Geometry: final body of the model. Coordinates: model frame, mm. Coordinates: 2 decimals unless noted, no trailing zeros. Order: outer loops, then holes, each group sorted by start corner. A loop starts at its lowest first (then second) coordinate and runs counter-clockwise, first axis right, second up. Notation, with made-up numbers: (31.25, 29) -> (62.25, 29) arc R24 ccw to (62.25, 39) -> close; hole circle Ø7 at (87, 58). An arc over 180 degrees is marked (long way). Answer in a Markdown table with one row per item. Add a question column.
1) Contact query for flat-ended pins moving along their axis: P1, Ø3, axis at x = -1.5, z = 134.5, coming from the +Y side; P2, Ø5, axis at x = -1, z = 131, coming from the -Y side; P3, Ø3, axis at x = 0, z = -23, coming from the -Y side; P4, Ø4, axis at x = 2.5, y = 10.5, coming from the +Z side. Output: stop coordinate, or through.
2) Ray query, line 1 (Y direction, x = 0, z = -0.25); line 2 (X direction, y = 22, z = 58.5); line 3 (Y direction, x = 0, z = 117.5). Return the intervals inside material, ascending. Write a range as from..to.
3) Section query A-A on z = 84. Return the cut outline in (x, y).
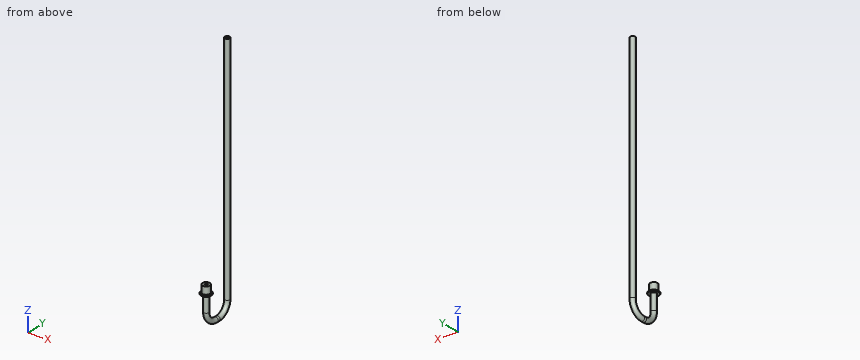
```python
from build123d import *

# Parameters (mm, degrees)
SKETCH1_R           = 4.25
BOSS_EXTRUDE1_DEPTH = 1
SKETCH2_R           = 3
BOSS_EXTRUDE2_DEPTH = 6
SKETCH3_R           = 2
CUT_EXTRUDE1_DEPTH  = 10.226321044
CHAMFER1_SIZE       = 0.2
SKETCH4_R           = 2
SKETCH4_R_2         = 1


with BuildPart() as part:
    # Sketch1 → Boss-Extrude1 (new body)
    with BuildSketch(Plane.XY):
        Circle(SKETCH1_R)
    extrude(amount=BOSS_EXTRUDE1_DEPTH)

    # Sketch2 → Boss-Extrude2 (add)
    with BuildSketch(Plane.XY.offset(1)):
        Circle(SKETCH2_R)
    extrude(amount=BOSS_EXTRUDE2_DEPTH)

    # Sketch3 → Cut-Extrude1 (cut, through all)
    with BuildSketch(Plane(origin=(0, 0, 0), x_dir=(-1, 0, 0), z_dir=(0, 0, -1))):
        Circle(SKETCH3_R)
    extrude(amount=-CUT_EXTRUDE1_DEPTH, mode=Mode.SUBTRACT)

    # Chamfer1
    chamfer1_edges = [part.edges().sort_by_distance(p)[0] for p in [
        (2, 0, 0),
        (-4.25, 0, 0),
        (-4.25, 0, 1),
    ]]
    chamfer(chamfer1_edges, length=CHAMFER1_SIZE)

    # Sweep1: sweep along a path in Sketch5
    with BuildLine(Plane(origin=(0, 0, 0), x_dir=(0, 0, -1), z_dir=(1, 0, 0))) as sweep1_path:
        Line((-7, 0), (13, 0))
        ThreePointArc((13, 0), (20.071067812, 2.928932188), (23, 10))
        Line((23, 10), (23, 12))
        ThreePointArc((23, 12), (20.071067812, 19.071067812), (13, 22))
        Line((13, 22), (-177, 22))
    # Sketch4 → Sweep1 (sweep)
    with BuildSketch(Plane.XY.offset(7)):
        Circle(SKETCH4_R)
        Circle(SKETCH4_R_2, mode=Mode.SUBTRACT)
    sweep(path=sweep1_path.line)


solid = part.part
```
Result:
| question | item | result |
|---|---|---|
| 1 | P1 | y = 24 |
| 1 | P2 | y = 20 |
| 1 | P3 | y = 1.53 |
| 1 | P4 | z = -21.06 |
| 2 | line 1 | -2..-1, 1..2, 20..21, 23..24 |
| 2 | line 2 | -2..-1, 1..2 |
| 2 | line 3 | 20..21, 23..24 |
| 3 | outline | circle Ø4 at (0, 22); hole circle Ø2 at (0, 22) |
